Design review of the part built by this model. Coordinates are the model's own, in mm. Give positions to 0.01 mm unless a question says otherwise; leave off trailing zeros. Loops run counter-clockwise (first coordinate to the right, second up) from the corner with the lowest first, then second, coordinate; pieces in that order, holes last. Notation, with made-up numbers: (-29, -16.5) - (-18, -16.5) arc R15 ccw to (-18, -5.5) - close; hole circle Ø9 at (32, -24.5). An arc over 180 degrees is marked (long way). Write each question's results on one line, items separated by ' | '.
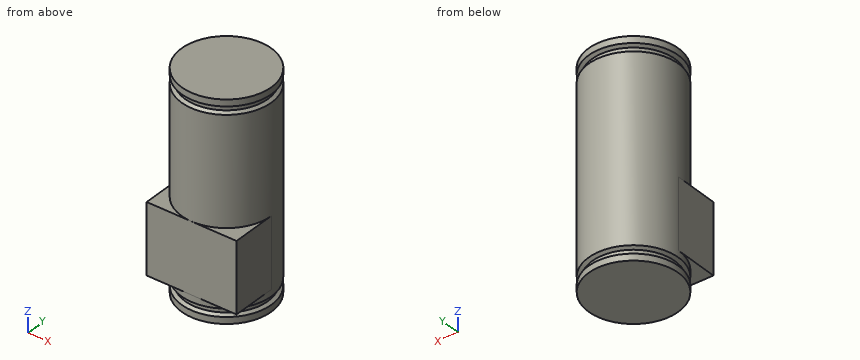
```python
from build123d import *

# Parameters (mm, degrees)
SKETCH010_R  = 16.875
PAD002_DEPTH = 8
PAD003_DEPTH = 26.3
SKETCH012_R  = 16.875
PAD004_DEPTH = 46


with BuildPart() as part:
    # Sketch010 → Pad002 (new body)
    with BuildSketch(Plane.XY):
        Circle(SKETCH010_R)
    extrude(amount=PAD002_DEPTH)

    # Sketch011 (on Face3 of Pad002) → Pad003 (join)
    with BuildSketch(Plane.XY.offset(8)):
        with BuildLine():
            Line((-16.875, 0), (-16.875, -16.875))
            Line((-16.875, -16.875), (16.875, -16.875))
            Line((16.875, -16.875), (16.875, 0))
            ThreePointArc((16.875, 0), (0, 16.875), (-16.875, 0))
        make_face()
    extrude(amount=PAD003_DEPTH)

    # Sketch012 (on Face6 of Pad003) → Pad004 (join)
    with BuildSketch(Plane.XY.offset(34.3)):
        Circle(SKETCH012_R)
    extrude(amount=PAD004_DEPTH)

    # Sketch013 → Groove (revolve, cut)
    with BuildSketch(Plane.XZ):
        Polygon((18.174038, 75.55), (18.174038, 77.05), (16.875, 77.8), (15.575962, 77.05), (15.575962, 75.55), (16.875, 74.8), align=None)
        Polygon((18.174038, 3.25), (18.174038, 4.75), (16.875, 5.5), (15.575962, 4.75), (15.575962, 3.25), (16.875, 2.5), align=None)
    revolve(axis=Axis((0, 0, 0), (0, 0, 1)), mode=Mode.SUBTRACT)


solid = part.part
```
Item 1: Wall thickness on probe 1 along Z at (x, y) = (9, 14); probe 2 along Z at (x, y) = (-14, 7.5); probe 3 along Y at (x, z) = (0, 53.5) (3 decimals): over which ranges is each line inside the solid? List them lowest first.
Output values:
probe 1: z = 0 to 2.63, 5.37 to 74.93, 77.67 to 80.3 | probe 2: z = 0 to 3.07, 4.93 to 75.37, 77.23 to 80.3 | probe 3: y = -16.875 to 16.875
Item 2: Clearance check with flat-ended pins moving along their axes: P1, Ø1, axis at x = -1.5, z = 65, coming from the +Y side; P2, Ø4, axis at y = -10, z = 50.5, coming from the -X side; P3, Ø1, axis at x = -2.5, z = 57, coming from the -Y side. State where each tip first meets the part, or that it passes through.
Output values:
P1: stops at y = 16.85 | P2: stops at x = -14.86 | P3: stops at y = -16.76
Item 3: We need section B-B on z = 30.5. Give the boundary of the cut face in (x, y) (3 decimals), then the cut area to 3 significant figures.
Output values:
outline: (-16.875, -16.875) - (16.875, -16.875) - (16.875, 0) arc R16.875 ccw to (-16.875, 0) - close | area: 1,020 mm²
Item 4: We need section A-A on z = 6.5. Give the boundary of the cut face in (x, y) (3 decimals), then the cut area to 3 significant figures.
Output values:
outline: circle Ø33.75 at (0, 0) | area: 895 mm²
